Design review of the part built by this model. Coordinates are the model's own, in mm. Face numbers are marked on the shaded views. Give positions to 0.01 mm unless a question says otherwise; leave off trailing zeros. Write each loop counter-clockwise with the first axis right and the second up, starting at its lowest first coordinate (ties: lowest second). Pieces come first, ordered by that corner, then holes. Notation, with made-up numbers: M -33,0.5 L -28,0.5 A23 ccw -28,28.5 Z; hole C 38,-38.5 d4. An arc over 180 degrees is marked long. One line per item, written item: value. Start each with the question number.
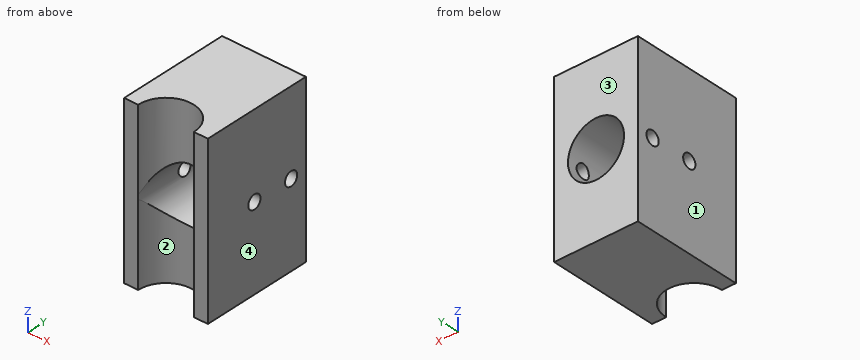
```python
from build123d import *

# Parameters (mm, degrees)
SKETCH1_W           = 38.1
SKETCH1_H           = 50.8
BOSS_EXTRUDE1_DEPTH = 76.2
SKETCH5_R           = 12.7
CUT_EXTRUDE3_DEPTH  = 77.2
SKETCH6_R           = 12.7635
CUT_EXTRUDE4_DEPTH  = 50.8
SKETCH7_R           = 3.175
CUT_EXTRUDE5_DEPTH  = 39.1


with BuildPart() as part:
    # Sketch1 → Boss-Extrude1 (new body)
    with BuildSketch(Plane.XY):
        Rectangle(SKETCH1_W, SKETCH1_H)
    extrude(amount=BOSS_EXTRUDE1_DEPTH)

    # Sketch5 → Cut-Extrude3 (cut, through all)
    with BuildSketch(Plane(origin=(0, 0, 0), x_dir=(-1, 0, 0), z_dir=(0, 0, -1))):
        with Locations((0, -25.4)):
            Circle(SKETCH5_R)
    extrude(amount=-CUT_EXTRUDE3_DEPTH, mode=Mode.SUBTRACT)

    # Sketch6 → Cut-Extrude4 (cut)
    with BuildSketch(Plane(origin=(0, 25.4, 0), x_dir=(1, 0, 0), z_dir=(0, 1, 0))):
        with Locations((0, -38.1)):
            Circle(SKETCH6_R)
    extrude(amount=-CUT_EXTRUDE4_DEPTH, mode=Mode.SUBTRACT)

    # Sketch7 → Cut-Extrude5 (cut, through all)
    with BuildSketch(Plane(origin=(19.05, 0, 0), x_dir=(0, 0, -1), z_dir=(1, 0, 0))):
        with Locations((-38.1, 17.78)):
            Circle(SKETCH7_R)
        with Locations((-38.1, -1.27)):
            Circle(SKETCH7_R)
    extrude(amount=-CUT_EXTRUDE5_DEPTH, mode=Mode.SUBTRACT)


solid = part.part
```
Q1. Take a section at A-A, the plane x = 0. Give the boundary of the cut face in (y, z).
Q2. Wall thickness on line 1 (Y direction, x = 17, z = 38); line 2 (Z direction, x = -14.25, y = -1.27) (3 decimals); line 3 (X direction, y = 13.5, z = 38.1): over which ranges is each line inside the solid? List them lowest first. Write a range as from..to.
Q3. Take a section at D-D, the plane y = 5. Give the boundary of the cut face in (x, z), then the cut area to 3 significant figures.
Q4. The part is to be moulded in two halves that separate along X. For the marked faces 1, 2, 3 and 4, say which applies: pulls with the +X half, pulls with the -X half, needs draft (parallel to the pull), parting line crosses it, or undercut.
Q5. Take a section at B-B, the plane z = 38.1. State how many separate pieces and enclosed holes the cut face has, then the cut area to 3 significant figures.
Q6. For P1, Ø5, axis at x = -0.5, z = 18.5, coming from the -Y side; P2, Ø4, axis at y = 17.78, z = 38.1, coming from the -X side; P3, Ø5, axis at x = 6, z = 60, coming from the -Y side, all flat-tipped, find the tip position at first contact; note any pin that passes through.
Results list:
1. outline: M -12.7,0 L 25.4,0 L 25.4,25.34 L -12.7,25.34 Z; M -12.7,50.86 L 25.4,50.86 L 25.4,76.2 L -12.7,76.2 Z
2. line 1: y = -25.4..-4.44, 1.9..14.61, 20.95..25.4
2. line 2: z = 0..34.925, 41.275..76.2
2. line 3: x = -19.05..-12.76, 12.76..19.05
3. outline: M -19.05,0 L 19.05,0 L 19.05,76.2 L -19.05,76.2 Z; hole C 0,38.1 d25.53
3. area: 2,390 mm^2
4. face 1: pulls with the -X half
4. face 2: undercut
4. face 3: needs draft
4. face 4: pulls with the +X half
5. separate pieces: 6
5. enclosed holes: 0
5. area: 479 mm^2
6. P1: stops at y = -13.06
6. P2: passes through
6. P3: stops at y = -15.96
